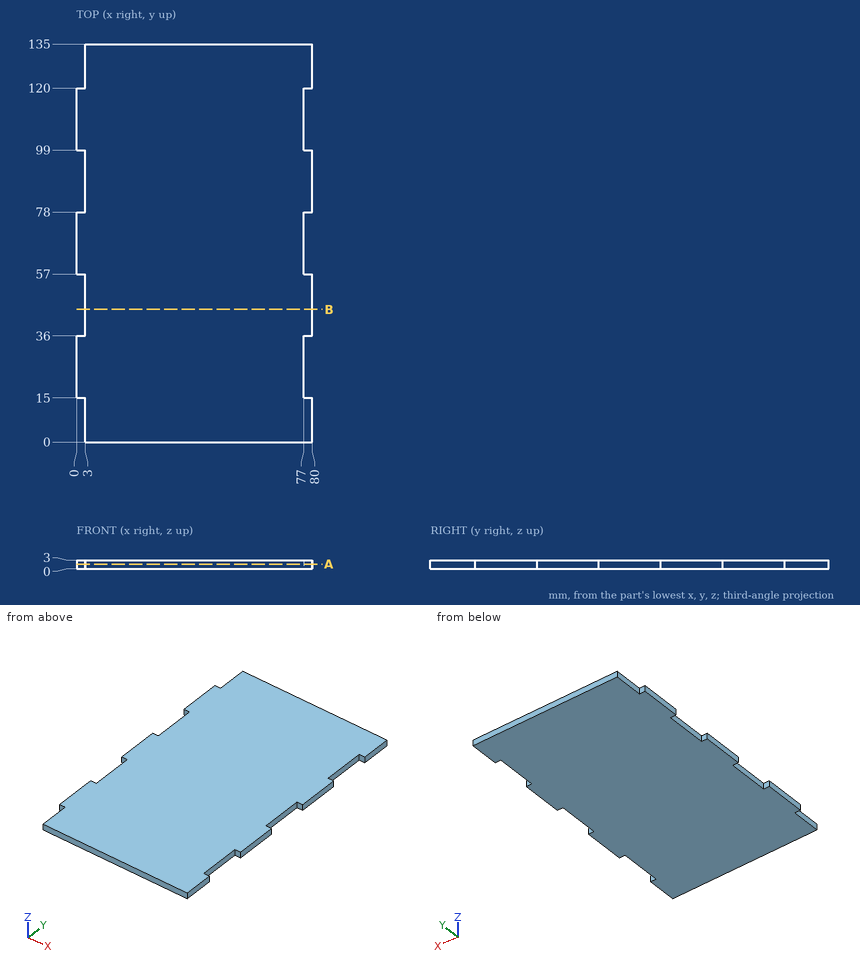
Geometry check sheet. Reference: drawing and pictorial views, mm from the part's lowest x, y, z. Round coordinates to 2 decimals unless told otherwise and drop trailing zeros. Order: outer loops, then holes, each group sorted by start corner. A loop starts at its lowest first (then second) coordinate and runs counter-clockwise, first axis right, second up. Notation, with made-up numbers: M 29,-23 L 36,-23 A26 ccw 36,0 Z; hole C -29,32.5 d8. An arc over 180 degrees is marked long. Answer in a Markdown table with one row per item.
(1) Scan lines: probe 1 along X at (y, z) = (16.5, 1.3); probe 2 along X at (y, z) = (126.5, 2.7). Record each from-to range of solid material in increasing order. Write a range as from..to.
Responses:
| item | result |
|---|---|
| probe 1 | x = 0..77 |
| probe 2 | x = 3..80 |
(2) Sectioned sample at A-A, the plane z = 1.6. Record the cut outline in (x, y), and give its area (3 significant figures).
Responses:
| item | result |
|---|---|
| outline | M 0,15 L 3,15 L 3,0 L 80,0 L 80,15 L 77,15 L 77,36 L 80,36 L 80,57 L 77,57 L 77,78 L 80,78 L 80,99 L 77,99 L 77,120 L 80,120 L 80,135 L 3,135 L 3,120 L 0,120 L 0,99 L 3,99 L 3,78 L 0,78 L 0,57 L 3,57 L 3,36 L 0,36 Z |
| area | 10,400 mm² |
(3) Sectioned sample at B-B, the plane y = 45. Record the cut outline in (x, z), and give its area (3 significant figures).
Responses:
| item | result |
|---|---|
| outline | M 3,0 L 80,0 L 80,3 L 3,3 Z |
| area | 231 mm² |
(4) Go/stop test with flat-tipped pins: P1, Ø0.9, axis at y = 90.5, z = 2, coming from the -X side; P2, Ø0.9, axis at x = 1, z = 2, coming from the -Y side; P3, Ø0.9, axis at x = 1.5, z = 1, coming from the +Y side. Record where each tip stops, or that it passes through.
Responses:
| item | result |
|---|---|
| P1 | stops at x = 3 |
| P2 | stops at y = 15 |
| P3 | stops at y = 120 |
